Answer from the drawing. Dimensions are ordinates in mm from the lowest x, y and z of the part. Give positions to 0.01 mm unless a question says otherwise; leave off trailing zeros. Loops run counter-clockwise (first coordinate to the right, second up) from the corner with the lowest first, then second, coordinate; pieces in that order, holes last.
Item 1: Each of these flat-tipped pins is pushed along its axis until it touches: pin 1 Ø1.5 at (x, z) = (109.5, 1) entering from -Y; pin 2 Ø0.9 at (x, z) = (32, 1.5) entering from +Y; pin 3 Ø1 at (x, y) = (99, 18) entering from -Z. Where does it stop, or does it pass through?
Item 2: Section D-D, the plane x = 163.5 is taken. Give the vertices of the cut face in (y, z).
Item 3: Section B-B, the plane y = 27.25 is taken. Give the vertices of the cut face in (x, z).
Item 4: Consider line 1 along X through (y, z) = (25.25, 1.3); line 2 along X through (y, z) = (12, 1.85); line 3 along Y through (x, z) = (76.5, 1.85). Determine where each line is inside the solid, lowest interval first.
Item 5: Section A-A, the plane y = 17.75 is taken. Give the vertices of the cut face in (x, z).
Item 6: Section C-C, the plane z = 2.45 is taken. Give the vertices of the cut face in (x, y), and give its area (3 significant figures).
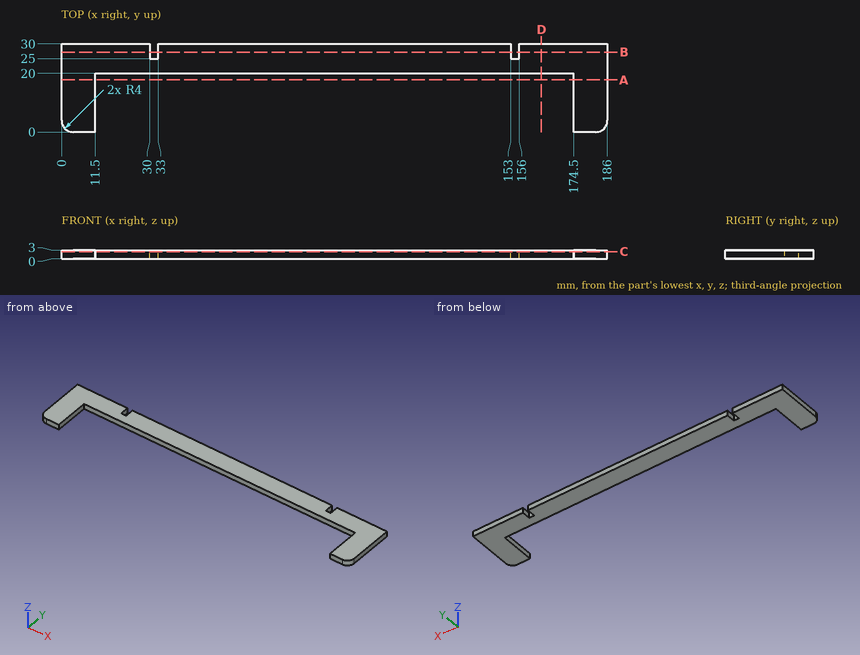
Worked answers:
1. pin 1: stops at y = 20
1. pin 2: stops at y = 25
1. pin 3: passes through
2. outline: (20, 0) - (30, 0) - (30, 3) - (20, 3) - close
3. outline: (0, 0) - (30, 0) - (30, 3) - (0, 3) - close; (33, 0) - (153, 0) - (153, 3) - (33, 3) - close; (156, 0) - (186, 0) - (186, 3) - (156, 3) - close
4. line 1: x = 0 to 30, 33 to 153, 156 to 186
4. line 2: x = 0 to 11.5, 174.5 to 186
4. line 3: y = 20 to 30
5. outline: (0, 0) - (11.5, 0) - (11.5, 3) - (0, 3) - close; (174.5, 0) - (186, 0) - (186, 3) - (174.5, 3) - close
6. outline: (0, 4) arc R4 ccw to (4, 0) - (11.5, 0) - (11.5, 20) - (174.5, 20) - (174.5, 0) - (182, 0) arc R4 ccw to (186, 4) - (186, 30) - (156, 30) - (156, 25) - (153, 25) - (153, 30) - (33, 30) - (33, 25) - (30, 25) - (30, 30) - (0, 30) - close
6. area: 2,280 mm2
